Check sheet for the modelled part. Datum: model origin and axes. Units: mm. A direction names the side the tool comes from. Give positions to 0.01 mm unless a question says otherwise; leave off trailing zeros. Order: outer loops, then holes, each group sorted by start corner. A loop starts at its lowest first (then second) coordinate and runs counter-clockwise, first axis right, second up. Notation, with made-up numbers: M -8,82 L 50,82 A36 ccw 50,120 Z; hole C 73,13 d1. An arc over 180 degrees is marked long. Answer in a Markdown table with one row per item. Add a question column.
from build123d import *

# Parameters (mm, degrees)
SALIENTE_EXTRUIR1_DEPTH = 6
CORTAR_EXTRUIR1_REACH   = 8
CROQUIS2_R              = 5.3
CROQUIS2_R_2            = 1.8
CROQUIS3_R              = 4
CROQUIS3_R_2            = 2.910883151
CROQUIS3_R_3            = 2.97880362
CORTAR_EXTRUIR2_DEPTH   = 4


with BuildPart() as part:
    # Croquis1 → Saliente-Extruir1 (new body)
    with BuildSketch(Plane(origin=(0, 0, 0), x_dir=(1, 0, 0), z_dir=(0, 1, 0))):
        Polygon((-50, 10.783872382), (-30.783872382, 30), (30.783872382, 30), (50, 10.783872382), (50, -10.783872382), (30.783872382, -30), (-30.783872382, -30), (-50, -10.783872382), align=None)
    extrude(amount=SALIENTE_EXTRUIR1_DEPTH)

    # Croquis2 → Cortar-Extruir1 (cut, up to next)
    with BuildSketch(Plane(origin=(0, 6, 0), x_dir=(1, 0, 0), z_dir=(0, 1, 0)), mode=Mode.PRIVATE) as cortar_extruir1_sk1:
        Circle(CROQUIS2_R)
    cortar_extruir1_tool1 = extrude(cortar_extruir1_sk1.sketch, amount=-CORTAR_EXTRUIR1_REACH, mode=Mode.PRIVATE) & part.part
    add(cortar_extruir1_tool1.solids().sort_by_distance((0, 6, 0))[0], mode=Mode.SUBTRACT)
    # Croquis2 → Cortar-Extruir1 (cut, up to next)
    with BuildSketch(Plane(origin=(0, 6, 0), x_dir=(1, 0, 0), z_dir=(0, 1, 0)), mode=Mode.PRIVATE) as cortar_extruir1_sk2:
        with Locations((-7.424621202, -7.424621202)):
            Circle(CROQUIS2_R_2)
    cortar_extruir1_tool2 = extrude(cortar_extruir1_sk2.sketch, amount=-CORTAR_EXTRUIR1_REACH, mode=Mode.PRIVATE) & part.part
    add(cortar_extruir1_tool2.solids().sort_by_distance((-7.424621, 6, 7.424621))[0], mode=Mode.SUBTRACT)
    # Croquis2 → Cortar-Extruir1 (cut, up to next)
    with BuildSketch(Plane(origin=(0, 6, 0), x_dir=(1, 0, 0), z_dir=(0, 1, 0)), mode=Mode.PRIVATE) as cortar_extruir1_sk3:
        with Locations((-7.827733398, 7.357422898)):
            Circle(CROQUIS2_R_2)
    cortar_extruir1_tool3 = extrude(cortar_extruir1_sk3.sketch, amount=-CORTAR_EXTRUIR1_REACH, mode=Mode.PRIVATE) & part.part
    add(cortar_extruir1_tool3.solids().sort_by_distance((-7.827733, 6, -7.357423))[0], mode=Mode.SUBTRACT)
    # Croquis2 → Cortar-Extruir1 (cut, up to next)
    with BuildSketch(Plane(origin=(0, 6, 0), x_dir=(1, 0, 0), z_dir=(0, 1, 0)), mode=Mode.PRIVATE) as cortar_extruir1_sk4:
        with Locations((6.954310702, 7.760535094)):
            Circle(CROQUIS2_R_2)
    cortar_extruir1_tool4 = extrude(cortar_extruir1_sk4.sketch, amount=-CORTAR_EXTRUIR1_REACH, mode=Mode.PRIVATE) & part.part
    add(cortar_extruir1_tool4.solids().sort_by_distance((6.954311, 6, -7.760535))[0], mode=Mode.SUBTRACT)
    # Croquis2 → Cortar-Extruir1 (cut, up to next)
    with BuildSketch(Plane(origin=(0, 6, 0), x_dir=(1, 0, 0), z_dir=(0, 1, 0)), mode=Mode.PRIVATE) as cortar_extruir1_sk5:
        with Locations((7.357422898, -7.021509007)):
            Circle(CROQUIS2_R_2)
    cortar_extruir1_tool5 = extrude(cortar_extruir1_sk5.sketch, amount=-CORTAR_EXTRUIR1_REACH, mode=Mode.PRIVATE) & part.part
    add(cortar_extruir1_tool5.solids().sort_by_distance((7.357423, 6, 7.021509))[0], mode=Mode.SUBTRACT)

    # Croquis3 → Cortar-Extruir2 (cut)
    with BuildSketch(Plane.XZ):
        with Locations((7.357422898, 7.021509007)):
            Circle(CROQUIS3_R)
        with Locations((6.954310702, -7.760535094)):
            Circle(CROQUIS3_R_2)
        with Locations((-7.424621202, 7.424621202)):
            Circle(CROQUIS3_R_3)
        with Locations((-7.827733398, -7.357422898)):
            Circle(CROQUIS3_R)
    extrude(amount=-CORTAR_EXTRUIR2_DEPTH, mode=Mode.SUBTRACT)


solid = part.part
Q1. Cross-section at C-C (y = 2.2). Record the boundary of the cut face in (x, z).
Q2. Go/stop test with flat-tipped pins: pin 1 (2 mm diameter, centred on y = 3, z = -12.5, fed in from -X); pin 2 (1.5 mm diameter, centred on x = -38.5, y = 0.5, fed in from -Z); pin 3 (4 mm diameter, centred on x = 6.5, z = 7, fed in from -Y). Record where each tip stops, or that it passes through.
Q3. Cross-section at B-B (z = -1). Record the boundary of the cut face in (x, y), and give its area (3 significant figures).
Q4. Draft check along X on faces 3 (the flat face through (1, 6, 6)), 4 (the flat face through (8, 4, -6)), 5 (the flat face through (40.526, 2.958, 20.257)). Enter one of: pulls with the +X half, pulls with the -X half, needs draft (parallel to the pull), parting line crosses it, or undercut.
Q5. Tool access check on faces 1 (the cylindrical face through (9.074, 5.014, 6.481)), 2 (the flat face through (-10, 4, -7)). Record the directions out of +Z, -Z, +X, -X, +Y, -Y that give a thin tool (end or side, any length) a straight path to the whole face; none if there is none.
Q6. Cross-section at D-D (z = -23.5). Record the boundary of the cut face in (x, y), and give its area (3 significant figures).
Q7. Thickness scan on probe 1 along X at (y, z) = (3.55, -10); probe 2 along Z at (x, y) = (-7.5, 2.6); probe 3 along X at (y, z) = (1, 10.5). Record the ranges inside material, lowest first.
Q8. Cross-section at A-A (x = 0). Record the boundary of the cut face in (y, z), and give its area (3 significant figures).
Values follow:
| question | item | result |
|---|---|---|
| 1 | outline | M -50,-10.78 L -30.78,-30 L 30.78,-30 L 50,-10.78 L 50,10.78 L 30.78,30 L -30.78,30 L -50,10.78 Z; hole C -7.83,-7.36 d8; hole C -7.42,7.42 d5.96; hole C 0,0 d10.6; hole C 7.36,7.02 d8; hole C 6.95,-7.76 d5.82 |
| 2 | pin 1 | x = -49.28 |
| 2 | pin 2 | z = -23.03 |
| 2 | pin 3 | y = 4 |
| 3 | outline | M -50,0 L -5.2,0 L -5.2,6 L -50,6 Z; M 5.2,0 L 50,0 L 50,6 L 5.2,6 Z |
| 3 | area | 538 mm² |
| 4 | face 3 | needs draft |
| 4 | face 4 | undercut |
| 4 | face 5 | pulls with the +X half |
| 5 | face 1 | +Y, -Y |
| 5 | face 2 | -Y |
| 6 | outline | M -37.28,0 L 37.28,0 L 37.28,6 L -37.28,6 Z |
| 6 | area | 447 mm² |
| 7 | probe 1 | -50 to -10.83, -4.82 to 5.09, 8.81 to 50 |
| 7 | probe 2 | -30 to -11.34, -3.37 to 4.45, 10.4 to 30 |
| 7 | probe 3 | -50 to 5.38, 9.33 to 50 |
| 8 | outline | M 0,-30 L 6,-30 L 6,-5.3 L 0,-5.3 Z; M 0,5.3 L 6,5.3 L 6,30 L 0,30 Z |
| 8 | area | 296 mm² |
